Source: CAD feature listing. Evaluate the final solid. Frame: model axes, mm. A direction names the side the tool comes from. Give positions to 0.01 mm unless a question says otherwise; leave off trailing zeros. Write each loop counter-clockwise with the first axis right and the second up, starting at its lowest first coordinate (ties: lowest second). Pieces come first, ordered by that corner, then holes.
Autodesk Inventor part; units mm, degrees
ref_plane "YZ Plane" through (0, 0, 0) normal (1, 0, 0) x (0, 1, 0)
ref_plane "XZ Plane" through (0, 0, 0) normal (0, 1, 0) x (-1, 0, 0)
ref_plane "XY Plane" through (0, 0, 0) normal (0, 0, 1) x (1, 0, 0)
sketch "Block1_1" plane through (0, 0, 0) normal (0, 0, 1) x (1, 0, 0)
  circle A0 centre (47.029, 24.2723) radius 1.1
  circle A1 centre (75.029, 24.2723) radius 1.1
  line L0 (49.279, 30.4723) -> (72.779, 30.4723)
  line L1 (72.779, 30.4723) -> (72.779, 18.0723)
  line L2 (72.779, 18.0723) -> (49.279, 18.0723)
  line L3 (49.279, 18.0723) -> (49.279, 30.4723)
  line L4 (49.279, 30.4723) -> (44.779, 30.4723)
  line L5 (44.779, 30.4723) -> (44.779, 18.0723)
  line L6 (44.779, 18.0723) -> (49.279, 18.0723)
  line L7 (49.279, 18.0723) -> (49.279, 30.4723)
  line L8 (72.779, 30.4723) -> (77.279, 30.4723)
  line L9 (77.279, 30.4723) -> (77.279, 18.0723)
  line L10 (77.279, 18.0723) -> (72.779, 18.0723)
  line L11 (72.779, 18.0723) -> (72.779, 30.4723)
  line L12 (44.779, 24.2723) -> (77.279, 24.2723) construction
  line L13 (61.029, 30.4723) -> (61.029, 18.0723) construction
  line L14 (47.029, 30.4723) -> (47.029, 18.0723) construction
  line L15 (75.029, 30.4723) -> (75.029, 18.0723) construction
  line L16 (66.779, 30.4723) -> (66.779, 18.0723) construction
  point P0 (60.979, 24.0984)
  dimension "d2" = 23.5
  dimension "d3" = 12.4
  dimension "d4" = 4.5
  dimension "d5" = 4.5
  dimension "d6" = 2.2
  dimension "d7" = 2.2
  dimension "d8" = 2.25
  dimension "d9" = 6
sketch "Sketch1" plane through (0, 0, 0) normal (0, 0, 1) x (1, 0, 0)
  line L0 (-18.5, 20) -> (18.5, 20)
  line L1 (18.5, 20) -> (18.5, -20)
  line L2 (18.5, -20) -> (-18.5, -20)
  line L3 (-18.5, -20) -> (-18.5, 20)
  circle A0 centre (-14, 0) radius 1.1
  circle A1 centre (14, 0) radius 1.1
  line L4 (-11.75, 6.2) -> (11.75, 6.2)
  line L5 (11.75, 6.2) -> (11.75, -6.2)
  line L6 (11.75, -6.2) -> (-11.75, -6.2)
  line L7 (-11.75, -6.2) -> (-11.75, 6.2)
  line L8 (-11.75, 6.2) -> (-16.25, 6.2)
  line L9 (-16.25, 6.2) -> (-16.25, -6.2)
  line L10 (-16.25, -6.2) -> (-11.75, -6.2)
  line L11 (-11.75, -6.2) -> (-11.75, 6.2)
  line L12 (11.75, 6.2) -> (16.25, 6.2)
  line L13 (16.25, 6.2) -> (16.25, -6.2)
  line L14 (16.25, -6.2) -> (11.75, -6.2)
  line L15 (11.75, -6.2) -> (11.75, 6.2)
  line L16 (-16.25, 0) -> (16.25, 0) construction
  line L17 (0, 6.2) -> (0, -6.2) construction
  line L18 (-14, 6.2) -> (-14, -6.2) construction
  line L19 (14, 6.2) -> (14, -6.2) construction
  line L20 (5.75, 6.2) -> (5.75, -6.2) construction
  point P0 (0, 0)
  point P1 (18.5, 0)
  point P2 (0, 20)
  point P3 (0, 0)
  dimension "d0" = 37
  dimension "d1" = 40
extrude "Extrusion1" add sketch "Sketch1" along normal blind 3 contours L0 L1 L2 L3 | L7 L10 L9 L8 | L12 L13 L14 L5
properties part number "ServoHolderPlate"
1. Pull-direction query (X, two-part tool) for faces 3 (the flat face through (0, 6.2, 1)), 4 (the flat face through (18.5, 0, 1)), 5 (the flat face through (0, -6.2, 1)), 6 (the flat face through (0, 20, 1)); classes: pulls with the +X half, pulls with the -X half, needs draft (parallel to the pull), parting line crosses it, or undercut.
2. Section query B-B (x = 14). Return loops of the section in (y, z).
3. Access query for faces 1 (the flat face through (-11.75, 0, 1)), 2 (the flat face through (-18.5, 0, 1)). Directions: +Z, -Z, +X, -X, +Y, -Y. A direction counts if a zero-diameter tool reaches every point of the face in a straight line with its end or side. Return the directions, or none.
4. Section query A-A (y = 0). Return loops of the section in (x, z).
5. Section query C-C (z = 1.7). Return loops of the section in (x, y).
6. Line query: probe 1 along X at (y, z) = (-3, 0.45); probe 2 along Y at (x, z) = (-8, 0.45); probe 3 along Y at (x, z) = (14, 2.15). Output: solid intervals per line, ascending.
7. Section query D-D (x = 8). Return loops of the section in (y, z).
The answers:
1. face 3: undercut
1. face 4: pulls with the +X half
1. face 5: undercut
1. face 6: needs draft
2. outline: (-20, 0) - (-1.1, 0) - (-1.1, 3) - (-20, 3) - close; (1.1, 0) - (20, 0) - (20, 3) - (1.1, 3) - close
3. face 1: +Z, -Z
3. face 2: +Z, -Z, -X, +Y, -Y
4. outline: (-18.5, 0) - (-15.1, 0) - (-15.1, 3) - (-18.5, 3) - close; (-12.9, 0) - (-11.75, 0) - (-11.75, 3) - (-12.9, 3) - close; (11.75, 0) - (12.9, 0) - (12.9, 3) - (11.75, 3) - close; (15.1, 0) - (18.5, 0) - (18.5, 3) - (15.1, 3) - close
5. outline: (-18.5, -20) - (18.5, -20) - (18.5, 20) - (-18.5, 20) - close; hole circle Ø2.2 at (-14, 0); hole (-11.75, -6.2) - (11.75, -6.2) - (11.75, 6.2) - (-11.75, 6.2) - close; hole circle Ø2.2 at (14, 0)
6. probe 1: x = -18.5 to -11.75, 11.75 to 18.5
6. probe 2: y = -20 to -6.2, 6.2 to 20
6. probe 3: y = -20 to -1.1, 1.1 to 20
7. outline: (-20, 0) - (-6.2, 0) - (-6.2, 3) - (-20, 3) - close; (6.2, 0) - (20, 0) - (20, 3) - (6.2, 3) - close
